from build123d import *

# Parameters (mm, degrees)
EXTRUDE_1_DEPTH     = 48
CUT_EXTRUDE_START   = 2
SKETCH_2_W          = 14
SKETCH_2_H          = 40
CUT_EXTRUDE_1_DEPTH = 48
SKETCH_3_W          = 12
SKETCH_3_H          = 40
CUT_EXTRUDE_2_DEPTH = 38
SKETCH_4_R          = 1.8
CUT_EXTRUDE_3_DEPTH = 38


with BuildPart() as part:
    # 草图1 → 凸台-拉伸1 (new body)
    with BuildSketch(Plane.XY):
        Polygon((-24, 0), (-14, 0), (10, 40), (0, 40), align=None)
    extrude(amount=EXTRUDE_1_DEPTH)

    # 草图2 → 切除-拉伸1 (cut)
    with BuildSketch(Plane(origin=(0, 0, 0), x_dir=(1, 0, 0), z_dir=(0, 1, 0)).offset(CUT_EXTRUDE_START)):
        with Locations((-24, -24)):
            Rectangle(SKETCH_2_W, SKETCH_2_H)
    extrude(amount=CUT_EXTRUDE_1_DEPTH, mode=Mode.SUBTRACT)

    # 草图3 → 切除-拉伸2 (cut)
    with BuildSketch(Plane(origin=(0, 0, 0), x_dir=(1, 0, 0), z_dir=(0, 1, 0))):
        with Locations((10, -24)):
            Rectangle(SKETCH_3_W, SKETCH_3_H)
    extrude(amount=CUT_EXTRUDE_2_DEPTH, mode=Mode.SUBTRACT)

    # 草图4 → 切除-拉伸3 (cut)
    with BuildSketch(Plane(origin=(0, 2, 0), x_dir=(1, 0, 0), z_dir=(0, 1, 0))):
        with Locations(Location((-20.4, -9, 0), (0, 0, 270))):
            Circle(SKETCH_4_R)
        with Locations(Location((-20.4, -39, 0), (0, 0, 270))):
            Circle(SKETCH_4_R)
    extrude(amount=-CUT_EXTRUDE_3_DEPTH, mode=Mode.SUBTRACT)


solid = part.part
CAD build for the part. Positions are in the model's coordinates, mm. A direction names the side the tool comes from. Coordinates: 2 decimals unless noted, no trailing zeros. Loops run counter-clockwise (first coordinate to the right, second up) from the corner with the lowest first, then second, coordinate; pieces in that order, holes last. Notation, with made-up numbers: (33, -40) - (37, -40) arc R22 cw to (37, -10) - close; hole circle Ø1 at (13, -16). An arc over 180 degrees is marked (long way). Use one line per item in the form item = value. Start each with the question number.
1) Band-saw the part on D-D (z = 32.5). Give the cut face in (x, y), and give its area (3 significant figures).
2) Band-saw the part on A-A (x = -20.4). Give the cut face in (y, z).
3) Band-saw the part on B-B (z = 39). Give the cut face in (x, y), and give its area (3 significant figures).
4) Drill centre lines: L1, parallel to Z at x = -17.5, y = 10.5; L2, parallel to Y at x = 5, z = 18; L3, parallel to X at y = 1.35, z = 39. Where is each one in solid material? Low to high. Write a range as from..to.
5) Two-plate mould, pull along X, no slides. Class faces 4 (the face through (-21.997, 1.014, 39.831)), 5 (the face through (-22.157, 1.014, 8.61)), 6 (the face through (4, 34, 24)), 7 (the face through (5, 36, 4)): +X half, -X half, draft (parallel to the pull), parting line (faces both ways), or undercut.
6) Tool access for faces 1 (the face through (-20, 2, 24)), 2 (the face through (5, 36, 44)), 3 (the face through (-8, 20, 0)): list every direction of +Z, -Z, +X, -X, +Y, -Y with a clear straight run to the whole face (end or side of a thin tool).
7) Band-saw the part on C-C (y = 31). Give the cut face in (x, z), and give its area (3 significant figures).
8) Flat gauge pins, fed straight in: pin 1 (6 mm diameter, centred on x = -20.5, z = 19.5, fed in from +Y); pin 2 (3 mm diameter, centred on y = 7, z = 27.5, fed in from -X); pin 3 (5 mm diameter, centred on y = 18.5, z = 16, fed in from +X). Where does each tip first touch, or does it go through?
Check values:
q1.outline = (-24, 0) - (-14, 0) - (4, 30) - (4, 38) - (8.8, 38) - (10, 40) - (0, 40) - (-17, 11.67) - (-17, 2) - (-22.8, 2) - close
q1.area = 353 mm2
q2.outline = (0, 0) - (6, 0) - (6, 4) - (2, 4) - (2, 7.2) - (0, 7.2) - close; (0, 10.8) - (2, 10.8) - (2, 37.2) - (0, 37.2) - close; (0, 40.8) - (2, 40.8) - (2, 44) - (6, 44) - (6, 48) - (0, 48) - close
q3.outline = (-24, 0) - (-22.2, 0) - (-22.2, 2) - (-22.8, 2) - close; (-18.6, 0) - (-14, 0) - (4, 30) - (4, 38) - (8.8, 38) - (10, 40) - (0, 40) - (-17, 11.67) - (-17, 2) - (-18.6, 2) - close
q3.area = 346 mm2
q4.L1 = 0..4, 44..48
q4.L2 = 38..40
q4.L3 = -23.19..-22.2, -18.6..-13.19
q5.face_4 = undercut
q5.face_5 = undercut
q5.face_6 = +X half
q5.face_7 = draft
q6.face_1 = -X, +Y
q6.face_2 = +X, -Y
q6.face_3 = -Z, +X, -X, +Y, -Y
q7.outline = (-5.4, 0) - (4.6, 0) - (4.6, 4) - (4, 4) - (4, 44) - (4.6, 44) - (4.6, 48) - (-5.4, 48) - close
q7.area = 456 mm2
q8.pin_1 = 2
q8.pin_2 = -17
q8.pin_3 = -1.4
